```python
from build123d import *

# Parameters (mm, degrees)
CROQUIS1_W              = 50
CROQUIS1_H              = 117
SALIENTE_EXTRUIR1_DEPTH = 5
CROQUIS2_W              = 50
CROQUIS2_H              = 11.75
SALIENTE_EXTRUIR2_DEPTH = 20
CORTAR_EXTRUIR1_DEPTH   = 10
CROQUIS5_R              = 1
CORTAR_EXTRUIR3_DEPTH   = 118


with BuildPart() as part:
    # Croquis1 → Saliente-Extruir1 (new body)
    with BuildSketch(Plane(origin=(0, 0, 0), x_dir=(1, 0, 0), z_dir=(0, 1, 0))):
        Rectangle(CROQUIS1_W, CROQUIS1_H)
    extrude(amount=SALIENTE_EXTRUIR1_DEPTH)

    # Croquis2 → Saliente-Extruir2 (add)
    with BuildSketch(Plane(origin=(0, 5, 0), x_dir=(1, 0, 0), z_dir=(0, 1, 0))):
        with Locations((0, 52.625)):
            Rectangle(CROQUIS2_W, CROQUIS2_H)
        with Locations((0, -52.625)):
            Rectangle(CROQUIS2_W, CROQUIS2_H)
    extrude(amount=SALIENTE_EXTRUIR2_DEPTH)

    # Croquis3 → Cortar-Extruir1 (cut)
    with BuildSketch(Plane(origin=(0, 5, 0), x_dir=(1, 0, 0), z_dir=(0, 1, 0))):
        with BuildLine():
            Line((25, 17.5), (9, 17.5))
            ThreePointArc((9, 17.5), (3.343145751, 15.156854249), (1, 9.5))
            Line((1, 9.5), (1, -9.5))
            ThreePointArc((1, -9.5), (3.343145751, -15.156854249), (9, -17.5))
            Line((9, -17.5), (25, -17.5))
            Line((25, -17.5), (25, 17.5))
        make_face()
    extrude(amount=-CORTAR_EXTRUIR1_DEPTH, mode=Mode.SUBTRACT)

    # Croquis5 → Cortar-Extruir3 (cut, through all)
    with BuildSketch(Plane(origin=(0, 0, -58.5), x_dir=(-1, 0, 0), z_dir=(0, 0, -1))):
        with Locations((0, 15)):
            Circle(CROQUIS5_R)
    extrude(amount=-CORTAR_EXTRUIR3_DEPTH, mode=Mode.SUBTRACT)


solid = part.part
```
Geometry: final body of the model. Coordinates: model frame, mm. A direction names the side the tool comes from. Round coordinates to 2 decimals unless told otherwise and drop trailing zeros. Write each loop counter-clockwise with the first axis right and the second up, starting at its lowest first coordinate (ties: lowest second). Pieces come first, ordered by that corner, then holes. Notation, with made-up numbers: (-13, 89.5) -> (-2, 89.5) arc R32 cw to (-2, 121.5) -> close; hole circle Ø4 at (76.25, -9.75). An arc over 180 degrees is marked (long way). Return JSON: item names as keys, results as strings.
Q1. Section A-A on x = 17.5. Return the cut outline in (y, z), and give its area (3 significant figures).
From the geometry:
{"outline": "(0, -58.5) -> (25, -58.5) -> (25, -46.75) -> (5, -46.75) -> (5, -17.5) -> (0, -17.5) -> close; (0, 17.5) -> (5, 17.5) -> (5, 46.75) -> (25, 46.75) -> (25, 58.5) -> (0, 58.5) -> close", "area": "880 mm2"}
Q2. Section C-C on z = -6.5. Return the cut outline in (x, y).
From the geometry:
{"outline": "(-25, 0) -> (1, 0) -> (1, 5) -> (-25, 5) -> close"}
Q3. First-contact query: pin 1 Ø10 at (y, z) = (7, 0.5) entering from +X; pin 2 Ø25 at (x, z) = (-6, 21.5) entering from +Y. Flat tips, straight axial feed; report the tip coordinate or a pass-through.
From the geometry:
{"pin 1": "x = 1", "pin 2": "y = 5"}
Q4. Section B-B on y = 10. Return the cut outline in (x, z).
From the geometry:
{"outline": "(-25, -58.5) -> (25, -58.5) -> (25, -46.75) -> (-25, -46.75) -> close; (-25, 46.75) -> (25, 46.75) -> (25, 58.5) -> (-25, 58.5) -> close"}
Q5. Ray query, line 1 (Z direction, x = 16, y = 5.25); line 2 (Y direction, x = 0, z = 52); line 3 (Z direction, x = 21, y = 4.5). Return the intervals inside material, ascending.
From the geometry:
{"line 1": "-58.5 to -46.75, 46.75 to 58.5", "line 2": "0 to 14, 16 to 25", "line 3": "-58.5 to -17.5, 17.5 to 58.5"}
Q6. Mould query, pull axis Z, two halves, no side actions, for faces 1 (the flat face through (0, 17, 46.75)), 2 (the flat face through (0, 0, -1)), 3 (the flat face through (0, 12, 58.5)). Classes: +Z half, -Z half, draft (parallel to the pull), parting line (faces both ways), or undercut.
From the geometry:
{"face 1": "undercut", "face 2": "draft", "face 3": "+Z half"}
Q7. Section D-D on z = 23. Return the cut outline in (x, y).
From the geometry:
{"outline": "(-25, 0) -> (25, 0) -> (25, 5) -> (-25, 5) -> close"}
Q8. Set-up query: faces 4 (the flat face through (0, 25, 53)), 5 (the flat face through (0, 17, -46.75)), 6 (the flat face through (17, 3, -17.5)). Return all of +Z, -Z, +X, -X, +Y, -Y with unobstructed straight access to the full face (end or side cutting, diameter ignored); none if empty.
From the geometry:
{"face 4": "+Z, -Z, +X, -X, +Y", "face 5": "+X, -X, +Y", "face 6": "+X, +Y, -Y"}
